```python
from build123d import *

# Parameters (mm, degrees)
F1_DEPTH = 11
F2_SIZE  = 5
F4_ANGLE = -90
F5_W     = 3
F5_H     = 3
F6_DEPTH = 80.001
F7_W     = 3
F7_H     = 3
F8_DEPTH = 25


with BuildPart() as f1:
    # F0 (on Front) → F1 (new body)
    with BuildSketch(Plane.XZ):
        Polygon((-40, 40), (-40, 0), (40, 0), (40, 40), (37, 40), (37, 3), (-37, 3), (-37, 40), align=None)
    extrude(amount=F1_DEPTH)

    # F2
    f2_edges = [f1.edges().sort_by_distance(p)[0] for p in [
        (-37, -5.5, 3),
        (37, -5.5, 3),
    ]]
    chamfer(f2_edges, length=F2_SIZE)


with BuildPart() as f1_1:
    # F4: moved
    add(f1.part.rotate(Axis((33.50826, 0, 0), (1, 0, 0)), F4_ANGLE))

    # F5 (on face) → F6 (cut, through all)
    with BuildSketch(Plane.YZ.offset(40)):
        with Locations((11.5, 5.5)):
            Rectangle(F5_W, F5_H)
        with Locations((31.5, 5.5)):
            Rectangle(F5_W, F5_H)
    extrude(amount=-F6_DEPTH, mode=Mode.SUBTRACT)

    # F7 (on face) → F8 (cut)
    with BuildSketch(Plane.XZ):
        with Locations((-28.5, 5.5)):
            Rectangle(F7_W, F7_H)
        with Locations((28.5, 5.5)):
            Rectangle(F7_W, F7_H)
    extrude(amount=-F8_DEPTH, mode=Mode.SUBTRACT)


solid = f1_1.part
```
Design review of the part built by this model. Coordinates are the model's own, in mm. A direction names the side the tool comes from. Coordinates: 2 decimals unless noted, no trailing zeros. Order: outer loops, then holes, each group sorted by start corner. A loop starts at its lowest first (then second) coordinate and runs counter-clockwise, first axis right, second up. Notation, with made-up numbers: (63.25, 77.5) - (74.25, 77.5) arc R15 ccw to (74.25, 95.5) - close; hole circle Ø5 at (49, -24). An arc over 180 degrees is marked (long way). Answer in a Markdown table with one row per item.
(1) Wall thickness on line 1 along X through (y, z) = (37, 1.75); line 2 along Y through (x, z) = (-2.5, 9.75); line 3 along X through (y, z) = (4, 5.5): over which ranges is each line inside the solid? List them lowest first. Write a range as from..to.
Checked values:
| item | result |
|---|---|
| line 1 | -40..-37, 37..40 |
| line 2 | 0..3 |
| line 3 | -40..-33, 33..40 |
(2) For faces 3 (the flat face through (37, 24, 5)), 4 (the flat face through (-1, 0, 5)), 5 (the flat face through (-38, 40, 5)), 6 (the flat face through (-29, 1, 4)), 7 (the flat face through (-38, 11, 4)), list the 3-axis set-ups (+Z, -Z, +X, -X, +Y, -Y) from which the entire face can be reached by the end or side of a thin tool; tool diameter is ignored.
Checked values:
| item | result |
|---|---|
| face 3 | +Z, -Z, +Y |
| face 4 | +Z, -Z, +X, -X, -Y |
| face 5 | +Z, -Z, +X, -X, +Y |
| face 6 | +Y, -Y |
| face 7 | +X, -X |
(3) Consider section A-A on y = 17. State the section outline as (x, z) points.
Checked values:
| item | result |
|---|---|
| outline | (-40, 0) - (-37, 0) - (-37, 11) - (-40, 11) - close; (37, 0) - (40, 0) - (40, 11) - (37, 11) - close |
(4) Clearance check with a flat-ended pin moving along its axis: pin 1 (6 mm diameter, centred on x = 23.5, z = 8.5, fed in from +Y). State where the tip first meets the part, or that it passes through.
Checked values:
| item | result |
|---|---|
| pin 1 | y = 3 |
(5) Consider section C-C on x = -34.5. State the section outline as (y, z) points, plus the area to 3 significant figures.
Checked values:
| item | result |
|---|---|
| outline | (0, 0) - (5.5, 0) - (5.5, 11) - (0, 11) - close |
| area | 60.5 mm^2 |
(6) Consider section D-D on x = -4. State the section outline as (y, z) points, plus the area to 3 significant figures.
Checked values:
| item | result |
|---|---|
| outline | (0, 0) - (3, 0) - (3, 11) - (0, 11) - close |
| area | 33.0 mm^2 |
(7) Consider section B-B on z = 2.25. State the section outline as (x, y) points.
Checked values:
| item | result |
|---|---|
| outline | (-40, 0) - (40, 0) - (40, 40) - (37, 40) - (37, 8) - (32, 3) - (-32, 3) - (-37, 8) - (-37, 40) - (-40, 40) - close |
(8) The part is to be moulded in two halves that separate along Z. For faces 1 (the flat face through (0, 3, 5)), 2 (the flat face through (-38, 10, 5)), say which applies: released by +Z, released by -Z, zero draft, split by the parting line, or undercut.
Checked values:
| item | result |
|---|---|
| face 1 | zero draft |
| face 2 | undercut |
